from build123d import *

# Parameters (mm, degrees)
F0_W     = 304.8
F0_H     = 152.4
F1_DEPTH = 5.207
F2_R     = 5.08
F3_R     = 4.8895
F4_DEPTH = 5.208
F5_R     = 11.1125
F6_DEPTH = 5.208


with BuildPart() as f1:
    # F0 (on Top) → F1 (new body)
    with BuildSketch(Plane.XY):
        Rectangle(F0_W, F0_H)
    extrude(amount=F1_DEPTH)

    # F2
    f2_edges = [f1.edges().sort_by_distance(p)[0] for p in [
        (-152.4, 76.2, 2.6035),
        (-152.4, -76.2, 2.6035),
        (152.4, 76.2, 2.6035),
        (152.4, -76.2, 2.6035),
    ]]
    fillet(f2_edges, radius=F2_R)

    # F3 (on face) → F4 (cut, through all)
    with BuildSketch(Plane.XY.offset(5.207)):
        with Locations((-144.3355, 68.1355)):
            Circle(F3_R)
        with Locations((-144.3355, -68.1355)):
            Circle(F3_R)
        with Locations((144.3355, 68.1355)):
            Circle(F3_R)
        with Locations((144.3355, -68.1355)):
            Circle(F3_R)
    extrude(amount=-F4_DEPTH, mode=Mode.SUBTRACT)

    # F5 (on face) → F6 (cut, through all)
    with BuildSketch(Plane.XY.offset(5.207)):
        with Locations((-106.3625, -52.3875)):
            Circle(F5_R)
        with Locations((-134.9375, -52.3875)):
            Circle(F5_R)
        with Locations((-134.9375, -17.4625)):
            Circle(F5_R)
        with Locations((-106.3625, -17.4625)):
            Circle(F5_R)
        with Locations((-134.9375, 17.4625)):
            Circle(F5_R)
        with Locations((-106.3625, 17.4625)):
            Circle(F5_R)
        with Locations((-134.9375, 52.3875)):
            Circle(F5_R)
        with Locations((-106.3625, 52.3875)):
            Circle(F5_R)
    extrude(amount=-F6_DEPTH, mode=Mode.SUBTRACT)


solid = f1.part
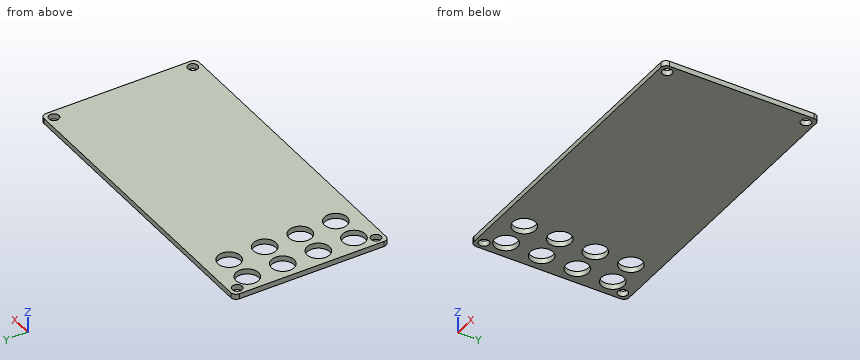
Model file for the job. Use its own axes, mm. Give positions to 0.01 mm unless a question says otherwise; leave off trailing zeros. Order: outer loops, then holes, each group sorted by start corner. A loop starts at its lowest first (then second) coordinate and runs counter-clockwise, first axis right, second up. Notation, with made-up numbers: M 40,-30 L 89,-30 A19 cw 89,-19 Z; hole C -31.75,-1 d9. An arc over 180 degrees is marked long. Put each result on its own line as item: value. Start each with the question number.
(1) Pin check, flat tips, straight feed: pin 1 Ø13.5 at (x, y) = (-106.36, 52.39) entering from -Z; pin 2 Ø10 at (x, y) = (-95, 19) entering from -Z. Stop position of each tip, or through.
(2) Drill centre lines: L1, parallel to X at y = 67.5, z = 0.45; L2, parallel to X at y = -25, z = 4.05; L3, parallel to Y at x = 140, z = 0.5. Where is each one in solid material? Low to high. Write a range as [from, to].
(3) Band-saw the part on C-C on y = 60. Give the cut face in (x, z).
(4) Band-saw the part on A-A on z = 0.9. Count the separate pieces of the cut face and the enclosed holes in it, then the cut area to 3 significant figures.
(5) Band-saw the part on B-B on y = -24. Give the cut face in (x, z), then the cut area to 3 significant figures.
Results below:
1. pin 1: passes through
1. pin 2: stops at z = 0
2. L1: x = [-152.4, -149.18], [-139.49, 139.49], [149.18, 152.4]
2. L2: x = [-152.4, -143.1], [-126.77, -114.53], [-98.2, 152.4]
2. L3: y = [-76.2, -70.4], [-65.87, 65.87], [70.4, 76.2]
3. outline: M -152.4,0 L -143.03,0 L -143.03,5.21 L -152.4,5.21 Z; M -126.84,0 L -114.46,0 L -114.46,5.21 L -126.84,5.21 Z; M -98.27,0 L 152.4,0 L 152.4,5.21 L -98.27,5.21 Z
4. separate pieces: 1
4. enclosed holes: 12
4. area: 43,000 mm2
5. outline: M -152.4,0 L -143.92,0 L -143.92,5.21 L -152.4,5.21 Z; M -125.95,0 L -115.35,0 L -115.35,5.21 L -125.95,5.21 Z; M -97.38,0 L 152.4,0 L 152.4,5.21 L -97.38,5.21 Z
5. area: 1,400 mm2
